Source: CAD feature listing. Evaluate the final solid. Frame: model axes, mm. Round coordinates to 2 decimals unless told otherwise and drop trailing zeros. One line per question, with ' | ' between items.
from build123d import *

# Parameters (mm, degrees)
PATTERN_CIRCULAR_3_COUNT = 24
SKETCH_6_R               = 2.5
CUT_EXTRUDE_1_DEPTH      = 17
PATTERN_CIRCULAR_2_COUNT = 2


with BuildPart() as part:
    # Sketch 1 → Revolve 2 (revolve)
    with BuildSketch(Plane.XY):
        with BuildLine():
            Line((-24.45, 126.6), (-13.603939201, 126.6))
            ThreePointArc((-13.603939201, 126.6), (-12.65, 125.9), (-11.696060799, 126.6))
            Line((-11.696060799, 126.6), (-0.85, 126.6))
            Line((-0.85, 126.6), (-0.35, 126.1))
            Line((-0.35, 126.1), (-0.35, 111.2))
            Line((-0.35, 111.2), (-1.982719633, 111.2))
            Line((-1.982719633, 111.2), (-1, 108.5))
            Line((-1, 108.5), (-1.55, 108.299816371))
            Line((-1.55, 108.299816371), (-1.55, 100.7))
            ThreePointArc((-1.55, 100.7), (-1.696446609, 100.346446609), (-2.05, 100.2))
            Line((-2.05, 100.2), (-18.95, 100.2))
            Line((-18.95, 100.2), (-18.95, 102.25))
            Line((-18.95, 102.25), (-24.95, 102.25))
            Line((-24.95, 102.25), (-24.95, 126.1))
            Line((-24.95, 126.1), (-24.45, 126.6))
        make_face()
    revolve(axis=Axis((0, 0, 0), (-1, 0, 0)))

    # Sketch 2 → Hole Wizard M81 (revolve, cut)
    with BuildSketch(Plane(origin=(-0.35, 114.958031676, -15.134511988), x_dir=(0, 0, -1), z_dir=(0, 1, 0))):
        Polygon((0, 0), (0, 24.6), (4.6, 24.6), (4.3, 24.3), (4.3, 0.3), (4.6, 0), align=None)
    hole_wizard_m81 = revolve(axis=Axis((6, 114.958031676, -15.134511988), (-1, 0, 0)), mode=Mode.SUBTRACT)

    # Pattern Circular 3: Hole Wizard M81 ×24 about axis
    pattern_circular_3_axis = Axis((0, 0, 0), (1, 0, 0))
    for i in range(1, PATTERN_CIRCULAR_3_COUNT):
        add(hole_wizard_m81.rotate(pattern_circular_3_axis, i * 360 / PATTERN_CIRCULAR_3_COUNT), mode=Mode.SUBTRACT)

    # Sketch 6 → Cut-Extrude 1 (cut)
    with BuildSketch(Plane.XY.offset(126.6)):
        with Locations((1.35, 0)):
            Circle(SKETCH_6_R)
    cut_extrude_1 = extrude(amount=-CUT_EXTRUDE_1_DEPTH, mode=Mode.SUBTRACT)

    # Pattern Circular 2: Cut-Extrude 1 ×2 about axis
    pattern_circular_2_axis = Axis((-110.150658921, 0, 0), (1, 0, 0))
    for i in range(1, PATTERN_CIRCULAR_2_COUNT):
        add(cut_extrude_1.rotate(pattern_circular_2_axis, i * 360 / PATTERN_CIRCULAR_2_COUNT), mode=Mode.SUBTRACT)


solid = part.part
1. Mould query, pull axis Z, two halves, no side actions, for faces 1 (the flat face through (-0.35, 114, -1)), 2 (the cylindrical face through (-12.48, 44.56, -111.42)). Classes: released by +Z, released by -Z, zero draft, split by the parting line, or undercut.
Worked out:
face 1: zero draft | face 2: undercut
2. Contact query for flat-ended pins moving along their axis: P1, Ø1, axis at x = -11, y = -16, coming from the -Z side; P2, Ø3, axis at x = -4, z = -83.5, coming from the +Y side; P3, Ø1, axis at y = -63.5, z = -83.5, coming from the +X side. Output: stop coordinate, or through.
Worked out:
P1: stops at z = -125.65 | P2: stops at y = 96.45 | P3: stops at x = -1.55
3. Material intervals for probe 1 along Z at (x, y) = (-6, 16); probe 2 along Z at (x, y) = (-4.75, 67); probe 3 along Z at (x, y) = (-12.5, -113.5), sorted ascending.
Worked out:
probe 1: z = -125.58 to -119.17, -110.75 to -98.91, 98.91 to 110.75, 119.17 to 125.58 | probe 2: z = -107.42 to -94.36, -89.62 to -74.51, 74.51 to 89.62, 94.36 to 107.42 | probe 3: z = -54.51 to -19.18, -11.09 to 11.09, 19.18 to 54.51
